Autodesk Inventor part; units mm, degrees
ref_plane "YZ Plane" through (0, 0, 0) normal (1, 0, 0) x (0, 1, 0)
ref_plane "XZ Plane" through (0, 0, 0) normal (0, 1, 0) x (-1, 0, 0)
ref_plane "XY Plane" through (0, 0, 0) normal (0, 0, 1) x (1, 0, 0)
sketch "Sketch1" plane through (0, 0, 0) normal (0, 0, 1) x (1, 0, 0)
  circle A0 centre (0, 0) radius 18.8
  circle A1 centre (0, 0) radius 4.15
  circle A2 centre (11.4, 0) radius 1.7
  circle A3 centre (0, 11.4) radius 1.7
  circle A4 centre (-11.4, 0) radius 1.7
  circle A5 centre (0, -11.4) radius 1.7
  dimension "d2" = 37.6
  dimension "d3" = 8.3
  dimension "d6" = 3.4
  dimension "d7" = 11.4
  dimension "d10" = 360
extrude "Extrusion1" add sketch "Sketch1" along normal blind 3
sketch "Sketch2" plane through (0, 0, 3) normal (0, 0, 1) x (1, 0, 0)
  circle A0 centre (0, 0) radius 4.15
  circle A1 centre (0, -11.4) radius 1.7
  circle A2 centre (-11.4, 0) radius 1.7
  circle A3 centre (0, 11.4) radius 1.7
  circle A4 centre (11.4, 0) radius 1.7
  circle A5 centre (0, 0) radius 18.8
  circle A6 centre (11.4, 0) radius 2.35
  circle A7 centre (0, 11.4) radius 2.35
  circle A8 centre (-11.4, 0) radius 2.35
  circle A9 centre (0, -11.4) radius 2.35
  dimension "d12" = 4.7
  dimension "d15" = 360
extrude "Extrusion2" add sketch "Sketch2" along normal blind 4.4 contours A6 | A7 | A8 | A9
chamfer "Chamfer1" distance 0.5 angle 45 8 edges at (-18.8, 0, 3) (-18.8, 0, 0) (-4.15, 0, 3) (-4.15, 0, 0) (-1.7, -11.4, 0) (9.7, 0, 0) (-1.7, 11.4, 0) (-13.1, 0, 0)
chamfer "Chamfer2" distance 0.2 angle 45 8 edges at (-13.75, 0, 7.4) (-13.1, 0, 7.4) (-1.7, 11.4, 7.4) (-2.35, 11.4, 7.4) (9.7, 0, 7.4) (9.05, 0, 7.4) (-1.7, -11.4, 7.4) (-2.35, -11.4, 7.4)
properties part number "Gear_Base_11.4mmD_4x_4.7mmW_3mmH_4.4mmE"
The model under review builds one solid part; all positions refer to its coordinate system, in mm. A direction names the side the tool comes from. Coordinates: 2 decimals unless noted, no trailing zeros. Write each loop counter-clockwise with the first axis right and the second up, starting at its lowest first coordinate (ties: lowest second). Pieces come first, ordered by that corner, then holes. Notation, with made-up numbers: (51, -15.5) - (71, -15.5) arc R19 ccw to (71, 12.5) - close; hole circle Ø3 at (-9.75, -30.75). An arc over 180 degrees is marked (long way). Answer in a Markdown table with one row per item. Add a question column.
Q1. For faces 3 (the face through (-9.16, -0.71, 5.07)), 4 (the face through (-9.78, -0.51, 3.8)), list the 3-axis set-ups (+Z, -Z, +X, -X, +Y, -Y) from which the entire face can be reached by the end or side of a thin tool; tool diameter is ignored.
Q2. Draft analysis for pull direction X (two halves, no side actions). For faces 1 (the face through (-0.37, 13.06, 3.8)), 2 (the face through (-4.08, 18.35, 1.49)), state which applies: +X half, -X half, draft (parallel to the pull), parting line (faces both ways), or undercut.
Q3. Clearance check with flat-ended pins moving along their axes: pin 1 (2 mm diameter, centred on x = 14.5, z = 5.5, fed in from +Y); pin 2 (13.5 mm diameter, centred on x = 0, y = 0, fed in from +Z); pin 3 (2.5 mm diameter, centred on x = 0, y = -11.4, fed in from +Z); pin 4 (2 mm diameter, centred on x = 13.5, z = 4.5, fed in from -Y). State where each tip first meets the part, or that it passes through.
Q4. Consider section B-B on y = 0. Give the number of separate pieces and of enclosed holes in the cut face, then the cut area to 3 significant figures.
Q5. Consider section A-A on z = 5. Give the boundary of the cut face in (x, y).
Q6. To check wall thickness, follow line 1 along Z through (x, y) = (-12, 5); line 2 along Y through (x, z) = (11.5, 2.5); line 3 along X through (y, z) = (-3.5, 1.25). State the ranges of each line that lie inside material, in increasing order. Write a range as from..to.
Answers below:
| question | item | result |
|---|---|---|
| 1 | face 3 | +Z |
| 1 | face 4 | +Z, -Z |
| 2 | face 1 | undercut |
| 2 | face 2 | parting line |
| 3 | pin 1 | y = 1.05 |
| 3 | pin 2 | z = 3 |
| 3 | pin 3 | through |
| 3 | pin 4 | y = -2.08 |
| 4 | separate pieces | 4 |
| 4 | enclosed holes | 0 |
| 4 | area | 77.3 mm² |
| 5 | outline | circle Ø4.7 at (-11.4, 0); circle Ø4.7 at (0, -11.4); circle Ø4.7 at (0, 11.4); circle Ø4.7 at (11.4, 0); hole circle Ø3.4 at (-11.4, 0); hole circle Ø3.4 at (0, -11.4); hole circle Ø3.4 at (0, 11.4); hole circle Ø3.4 at (11.4, 0) |
| 6 | line 1 | 0..3 |
| 6 | line 2 | -14.87..-1.7, 1.7..14.87 |
| 6 | line 3 | -18.47..-2.23, 2.23..18.47 |
